Verification items for the finished model (mm, model axes). Face numbers are marked on the shaded views. A direction names the side the tool comes from. Give positions to 0.01 mm unless a question says otherwise; leave off trailing zeros. Order: outer loops, then holes, each group sorted by start corner. A loop starts at its lowest first (then second) coordinate and runs counter-clockwise, first axis right, second up. Notation, with made-up numbers: (26.25, -15.75) -> (45.25, -15.75) arc R18 ccw to (45.25, 15.25) -> close; hole circle Ø1 at (31.5, 20). An arc over 180 degrees is marked (long way). Return JSON: item names as keys, results as strings. Group by question number.
(1) Cross-section at D-D on y = 79.5. Enter the section's corners in (x, z), then the cut area to 3 significant figures.
(2) Cross-section at A-A on z = 0. Enter the section's corners in (x, y), then the cut area to 3 significant figures.
(3) Release check for a two-part mould opening along Z. For the marked faces 1, 2 and 3 record: pulls with the +Z half, pulls with the -Z half, needs draft (parallel to the pull), parting line crosses it, or undercut.
(4) Tool access check on the marked faces 4, 5 and 6. Record the directions out of +Z, -Z, +X, -X, +Y, -Y that give a thin tool (end or side, any length) a straight path to the whole face; none if there is none.
(5) Cross-section at C-C on y = 30. Enter the section's corners in (x, z), then the cut area to 3 significant figures.
(6) Thickness scan on line 1 along Y through (x, z) = (-5, 0); line 2 along Z through (x, y) = (-1, 30); line 3 along Y through (x, z) = (-8, -15). Record the ranges inside material, lowest first.
(7) Cross-section at B-B on x = 0. Enter the section's corners in (y, z), then the cut area to 3 significant figures.
(8) Depth check by flat-ended pin: pin 1 Ø2 at (y, z) = (76.5, 12) entering from +X; pin 2 Ø4 at (x, y) = (3.5, 26) entering from +Z; pin 3 Ø19.5 at (x, z) = (-1, 1) entering from -Y; pin 4 Ø6 at (x, y) = (-4, 35.5) entering from -Z. Enter the tip coordinate at first touch or a pass-through.
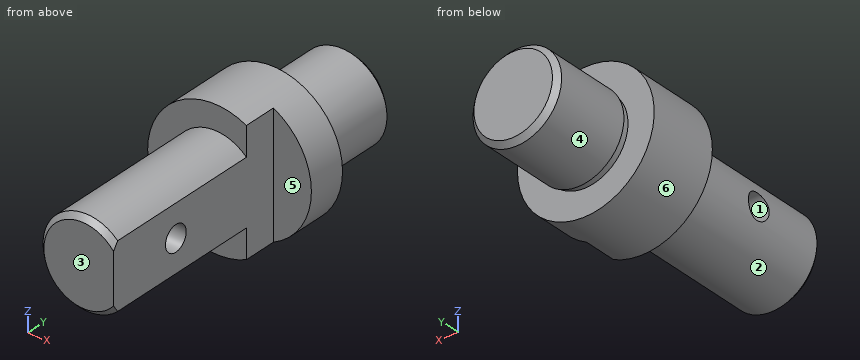
Autodesk Inventor part; units mm, degrees
ref_plane "Work Plane1" through (27, 64, 0) normal (1, 0, 0) x (0, 1, 0)
ref_plane "XZ Plane" through (0, 0, 0) normal (0, 1, 0) x (-1, 0, 0)
ref_plane "XY Plane" through (0, 0, 0) normal (0, 0, 1) x (1, 0, 0)
sketch "Sketch1" plane through (0, 0, 0) normal (0, 1, 0) x (-1, 0, 0)
  circle A0 centre (0, 0) radius 17.5
  dimension "d0" = 35
extrude "Extrusion1" add sketch "Sketch1" along normal blind 64
sketch "Sketch2" plane through (0, 64, 0) normal (0, 1, 0) x (1, 0, 0)
  circle A0 centre (0, 0) radius 27
  dimension "d3" = 54
extrude "Extrusion2" add sketch "Sketch2" along normal blind 28
sketch "Sketch3" plane through (0, 92, 0) normal (0, 1, 0) x (1, 0, 0)
  circle A0 centre (0, 0) radius 16.65
  dimension "d6" = 33.3
extrude "Extrusion3" add sketch "Sketch3" along normal blind 3
sketch "Sketch4" plane through (0, 95, 0) normal (0, 1, 0) x (1, 0, 0)
  circle A0 centre (0, 0) radius 16.65
  circle A1 centre (0, 0) radius 17.5
  dimension "d9" = 35
extrude "Extrusion4" add sketch "Sketch4" along normal blind 32 contours A0 | A1
ref_plane "Work Plane1" through (27, 64, 0) normal (1, 0, 0) x (0, 1, 0)
sketch "Sketch5" plane through (27, 64, 0) normal (1, 0, 0) x (0, 1, 0)
  line L0 (-64, -17.5) -> (-64, 17.5)
  line L1 (-64, -17.5) -> (-64, -50.6158)
  line L2 (-64, -50.6158) -> (13, -50.6158)
  line L3 (13, -50.6158) -> (-82.5223, -50.6158)
  line L4 (-82.5223, -50.6158) -> (-82.5223, 53.8814)
  line L5 (-82.5223, 53.8814) -> (13, 53.8814)
  line L6 (13, 53.8814) -> (13, -50.6158)
  point P0 (-64, 0)
  dimension "d12" = 77
extrude "Extrusion5" cut sketch "Sketch5" against normal blind 15
sketch "Sketch6" plane through (12, 64, 0) normal (1, 0, 0) x (0, 0, -1)
  line L0 (17.5, -64) -> (-17.5, -64)
  line L1 (-17.5, -64) -> (0, -64)
  line L2 (0, -64) -> (0, -34)
  line L3 (0, -34) -> (-17.5, -34)
  line L4 (-17.5, -34) -> (-17.5, -64)
  circle A0 centre (0, -34) radius 5
  point P0 (12.7377, -64)
  point P1 (-12.7377, -64)
  dimension "d15" = 30
  dimension "d16" = 10
extrude "Extrusion6" cut sketch "Sketch6" against normal through all contours A0 L3 L2 | L2 L3 A0
chamfer "Chamfer1" distance 2 angle 45 2 edges at (-17.5, 0, 0) (-17.5, 127, 0)
properties part number "MMAE 232 Assignment 1c-Nicholas Skiba" material "Aluminum 6061"
Verdict:
{
 "1": {"outline": "circle Ø54 at (0, 0)", "area": "2,290 mm²"},
 "2": {"outline": "(-27, 64) -> (-17.5, 64) -> (-17.5, 35) -> (12, 35) -> (12, 77) -> (27, 77) -> (27, 92) -> (16.65, 92) -> (16.65, 95) -> (17.5, 95) -> (17.5, 125) -> (15.5, 127) -> (-15.5, 127) -> (-17.5, 125) -> (-17.5, 95) -> (-16.65, 95) -> (-16.65, 92) -> (-27, 92) -> close; (-17.5, 2) -> (-15.5, 0) -> (12, 0) -> (12, 25) -> (-17.5, 25) -> close", "area": "4,120 mm²"},
 "3": {"face 1": "undercut", "face 2": "parting line crosses it", "face 3": "needs draft"},
 "4": {"face 4": "+Y", "face 5": "+Z, -Z, +X, -Y", "face 6": "+Y, -Y"},
 "5": {"outline": "(-16.77, -5) arc R17.5 ccw to (12, -12.74) -> (12, -5) -> close; (-16.77, 5) -> (12, 5) -> (12, 12.74) arc R17.5 ccw to start", "area": "573 mm²"},
 "6": {"line 1": "0 to 25, 35 to 127", "line 2": "-17.47 to -5, 5 to 17.47", "line 3": "1.5 to 92, 95 to 125.5"},
 "7": {"outline": "(0, -15.5) -> (2, -17.5) -> (64, -17.5) -> (64, -27) -> (92, -27) -> (92, -16.65) -> (95, -16.65) -> (95, -17.5) -> (125, -17.5) -> (127, -15.5) -> (127, 15.5) -> (125, 17.5) -> (95, 17.5) -> (95, 16.65) -> (92, 16.65) -> (92, 27) -> (64, 27) -> (64, 17.5) -> (2, 17.5) -> (0, 15.5) -> close; hole circle Ø10 at (30, 0)", "area": "4,890 mm²"},
 "8": {"pin 1": "x = 24.6", "pin 2": "z = 17.44", "pin 3": "y = 0", "pin 4": "z = -17.47"}
}
